Read the model definition and answer for the solid it produces. Units are mm, in the model's axes. A direction names the side the tool comes from. Coordinates: 2 decimals unless noted, no trailing zeros. Put each result on its own line as item: value.
from build123d import *

# Parameters (mm, degrees)
SKETCH1_W           = 63.5
SKETCH1_H           = 63.5
BOSS_EXTRUDE1_DEPTH = 1.5875
SKETCH2_W           = 57.15
SKETCH2_H           = 57.15
SKETCH2_W_2         = 56.35
SKETCH2_H_2         = 56.35
BOSS_EXTRUDE2_DEPTH = 1.5875
SKETCH3_R           = 9.525
BOSS_EXTRUDE4_DEPTH = 2.54
SKETCH5_R           = 3.6195
CUT_EXTRUDE2_DEPTH  = 46.090589442
SKETCH6_W           = 3.175
SKETCH6_H           = 3.429
CUT_EXTRUDE3_DEPTH  = 2.54
SKETCH7_R           = 3.175
BOSS_EXTRUDE5_DEPTH = 0.26


with BuildPart() as part:
    # Sketch1 → Boss-Extrude1 (new body)
    with BuildSketch(Plane.XY):
        Rectangle(SKETCH1_W, SKETCH1_H)
    extrude(amount=BOSS_EXTRUDE1_DEPTH)

    # Sketch2 → Boss-Extrude2 (add)
    with BuildSketch(Plane.XY.offset(1.5875)):
        Rectangle(SKETCH2_W, SKETCH2_H)
        Rectangle(SKETCH2_W_2, SKETCH2_H_2, mode=Mode.SUBTRACT)
    extrude(amount=BOSS_EXTRUDE2_DEPTH)

    # Sketch3 → Boss-Extrude4 (add)
    with BuildSketch(Plane.XY.offset(1.5875)):
        with Locations(Location((-15.875, -13.335, 0), (0, 0, 180))):
            Circle(SKETCH3_R)
        with Locations(Location((0, 14.16130657, 0), (0, 0, 180))):
            Circle(SKETCH3_R)
        with Locations(Location((15.875, -13.335, 0), (0, 0, 180))):
            Circle(SKETCH3_R)
    extrude(amount=BOSS_EXTRUDE4_DEPTH)

    # Sketch5 → Cut-Extrude2 (cut, through all)
    with BuildSketch(Plane.XY.offset(4.1275)):
        with Locations((0, 14.16130657)):
            Circle(SKETCH5_R)
        with Locations((15.875, -13.335)):
            Circle(SKETCH5_R)
        with Locations((-15.875, -13.335)):
            Circle(SKETCH5_R)
    extrude(amount=-CUT_EXTRUDE2_DEPTH, mode=Mode.SUBTRACT)

    # Sketch6 → Cut-Extrude3 (cut)
    with BuildSketch(Plane.XY.offset(4.1275)):
        with Locations((8.255, 14.16130657)):
            Rectangle(SKETCH6_W, SKETCH6_H)
        with Locations((-25.4, -13.335)):
            Rectangle(SKETCH6_W, SKETCH6_H)
        with Locations((7.62, -13.335)):
            Rectangle(SKETCH6_W, SKETCH6_H)
    extrude(amount=-CUT_EXTRUDE3_DEPTH, mode=Mode.SUBTRACT)

    # Sketch7 → Boss-Extrude5 (add)
    with BuildSketch(Plane(origin=(0, 0, 0), x_dir=(-1, 0, 0), z_dir=(0, 0, -1))):
        with Locations((31.75, -31.75)):
            Circle(SKETCH7_R)
        with Locations((-31.75, -31.75)):
            Circle(SKETCH7_R)
        with Locations((-31.75, 31.75)):
            Circle(SKETCH7_R)
        with Locations((31.75, 31.75)):
            Circle(SKETCH7_R)
    extrude(amount=-BOSS_EXTRUDE5_DEPTH)


solid = part.part
Q1. A tool of negligible diameter and unlimited length cuts with its end or side. For faces 1 (the face through (-9.517, 14.556, 2.84)), 2 (the face through (15.404, -9.746, 2.093)), 3 (the face through (0, -28.575, 2)), from which of +Z, -Z, +X, -X, +Y, -Y can it reach the whole face along a straight path? Write none if from no direction.
Answers below:
face 1: +Z
face 2: +Z, -Z
face 3: +Z, +X, -X, -Y
Q2. Consider line 1 along Y through (x, z) = (0, 2.45) (3 decimals); line 2 along X through (y, z) = (6, 2.55) (3 decimals); line 3 along Y through (x, z) = (18, 2.55) (3 decimals). Determine where each line is inside the solid, lowest interval first.
Answers below:
line 1: y = -28.575 to -28.175, 4.636 to 10.542, 17.781 to 23.686, 28.175 to 28.575
line 2: x = -28.575 to -28.175, -4.911 to 4.911, 28.175 to 28.575
line 3: y = -28.575 to -28.175, -22.62 to -16.265, -10.405 to -4.05, 28.175 to 28.575
Q3. Given pin 1 (0.8 mm diameter, centred on x = -9.5, z = 2.5, fed in from -Y) (3 decimals); pin 2 (1.7 mm diameter, centred on y = -11, z = 2, fed in from +X); pin 3 (1.3 mm diameter, centred on y = -13, z = 2.5, fed in from -X) (3 decimals); pin 4 (3 mm diameter, centred on x = 14.5, y = -13, fed in from -Z), each flat-ended and moving along its own axis, determine where each tip first touches the part or whether it passes through.
Answers below:
pin 1: stops at y = -28.575
pin 2: stops at x = 31.75
pin 3: stops at x = -28.575
pin 4: passes through
Q4. For a pull along Y with two mould halves and no side action, classify faces 4 (the face through (0, 28.175, 2)), 5 (the face through (0, -31.75, 1)), 6 (the face through (6.668, 14, 3)), 7 (the face through (-28.575, 0, 2)) as +Y half, -Y half, draft (parallel to the pull), parting line (faces both ways), or undercut.
Answers below:
face 4: undercut
face 5: -Y half
face 6: undercut
face 7: draft
